from build123d import *

# Parameters (mm, degrees)
PAD009_DEPTH    = 350
POCKET015_DEPTH = 22.001
PAD010_DEPTH    = 20
SKETCH031_R     = 1.5
POCKET016_DEPTH = 5
SKETCH032_R     = 1.5
POCKET017_DEPTH = 5
SKETCH033_R     = 1.5
POCKET018_DEPTH = 5
SKETCH035_R     = 1.5
POCKET020_DEPTH = 5
SKETCH071_R     = 1.5
POCKET047_DEPTH = 5


with BuildPart() as part:
    # Sketch028 (on Face2 of Binder006) → Pad009 (new body)
    with BuildSketch(Plane(origin=(0, -0.1, 0), x_dir=(-1, 0, 0), z_dir=(0, 1, 0))):
        Polygon((-627, -343.2), (-627, 133.2535631324), (-605.051890377, 134.7636902715), (-605.051890377, 132.7636902715), (-625, 131.2535631324), (-625, -341.2), (-605, -341.2), (-605, -343.2), align=None)
    extrude(amount=PAD009_DEPTH)

    # Sketch029 (on Face2 of Pad009) → Pocket015 (cut, through all)
    with BuildSketch(Plane.YZ.offset(627)):
        Polygon((-0.1, -203.2), (195.0232253156, 134.7636902715), (-0.1, 134.7636902715), align=None)
    extrude(amount=-POCKET015_DEPTH, mode=Mode.SUBTRACT)

    # Sketch030 (on Face9 of Pocket015) → Pad010 (join)
    with BuildSketch(Plane(origin=(625, 0, 0), x_dir=(0, -1, 0), z_dir=(-1, 0, 0))):
        Polygon((0.1, -341.2), (0.1, -203.2), (-192.9966545674, 131.2535631324), (-194.9966545674, 131.2535631324), (-1.9, -203.2), (-1.9, -341.2), align=None)
    extrude(amount=PAD010_DEPTH)

    # Sketch031 (on Face2 of Binder006) → Pocket016 (cut)
    with BuildSketch(Plane(origin=(0, -0.1, 0), x_dir=(-1, 0, 0), z_dir=(0, 1, 0))):
        with Locations((-615, -213.2)):
            Circle(SKETCH031_R)
        with Locations((-616.35879, -273.2)):
            Circle(SKETCH031_R)
        with Locations((-615, -333.2)):
            Circle(SKETCH031_R)
    extrude(amount=POCKET016_DEPTH, mode=Mode.SUBTRACT)

    # Sketch032 (on Face6 of Pocket016) → Pocket017 (cut)
    with BuildSketch(Plane(origin=(0, 87.9131353872, -50.7566197735), x_dir=(1, 0, 0), z_dir=(0, -0.8660256282, 0.4999996113))):
        with Locations((615, -166.026408)):
            Circle(SKETCH032_R)
        with Locations((615, 17.070397)):
            Circle(SKETCH032_R)
        with Locations((615, 113.6188)):
            Circle(SKETCH032_R)
        with Locations((615, 200.167202)):
            Circle(SKETCH032_R)
        with Locations((615, -74.478005)):
            Circle(SKETCH032_R)
    extrude(amount=-POCKET017_DEPTH, mode=Mode.SUBTRACT)

    # Sketch033 (on Face10 of Pocket017) → Pocket018 (cut)
    with BuildSketch(Plane.XY.offset(-341.2)):
        with Locations((615, 11.9)):
            Circle(SKETCH033_R)
        with Locations((615, 93.9)):
            Circle(SKETCH033_R)
        with Locations((615, 175.9)):
            Circle(SKETCH033_R)
        with Locations((615, 267.9)):
            Circle(SKETCH033_R)
        with Locations((615, 339.9)):
            Circle(SKETCH033_R)
    extrude(amount=-POCKET018_DEPTH, mode=Mode.SUBTRACT)

    # Sketch035 (on Face19 of Pocket018) → Pocket020 (cut)
    with BuildSketch(Plane(origin=(12.0794992713, 0, 175.5628167535), x_dir=(0.9976413465, 0, -0.0686421427), z_dir=(0.0686421427, 0, 0.9976413465))):
        with Locations((604.374314, 272.461613)):
            Circle(SKETCH035_R)
        with Locations((604.374314, 339.9)):
            Circle(SKETCH035_R)
        with Locations((604.374314, 205.023225)):
            Circle(SKETCH035_R)
    extrude(amount=-POCKET020_DEPTH, mode=Mode.SUBTRACT)

    # Sketch071 (on Face1 of Binder021) → Pocket047 (cut)
    with BuildSketch(Plane.YZ.offset(629)):
        with Locations((339.9, -213.170471)):
            Circle(SKETCH071_R)
        with Locations((257.904262, -213.170471)):
            Circle(SKETCH071_R)
        with Locations((175.908524, -213.170471)):
            Circle(SKETCH071_R)
        with Locations((93.912786, -213.170471)):
            Circle(SKETCH071_R)
        with Locations((11.917049, -213.170471)):
            Circle(SKETCH071_R)
    extrude(amount=-POCKET047_DEPTH, mode=Mode.SUBTRACT)


solid = part.part
Source: CAD feature listing. Evaluate the final solid. Frame: model axes, mm. A direction names the side the tool comes from. Coordinates: 2 decimals unless noted, no trailing zeros. Order: outer loops, then holes, each group sorted by start corner. A loop starts at its lowest first (then second) coordinate and runs counter-clockwise, first axis right, second up. Notation, with made-up numbers: M 7.25,15 L 37.25,15 A26 ccw 37.25,39 Z; hole C 20.25,61.25 d5. An arc over 180 degrees is marked long. Write each question's results on one line, items separated by ' | '. Start each with the question number.
1. Pin query (flat end, axial travel): pin 1 (2.5 mm diameter, centred on x = 615, y = 93.9, fed in from -Z); pin 2 (4 mm diameter, centred on y = 339.9, z = -213.17, fed in from -X); pin 3 (4 mm diameter, centred on x = 615, y = 267.9, fed in from -Z); pin 4 (1 mm diameter, centred on x = 610.5, y = 193.5, fed in from +Z). Return the tip coordinate at first contact, or that it passes through.
2. Section A-A, the plane y = 237. Return the cut outline in (x, z).
3. Section B-B, the plane z = -92.5. Return the cut outline in (x, y), then the cut area to 3 significant figures.
4. Reachability of faces 1 (the face through (615, 173, -341.2)), 2 (the face through (614, -0.1, -274)) from +Z, -Z, +X, -X, +Y, -Y: full face, straight path, thin tool, end or side. Return the list, or none.
5. Material intervals for L1, parallel to Y at x = 615, z = -342; L2, parallel to Z at x = 615, y = 1.1; L3, parallel to Z at x = 615, y = 258, sorted ascending.
6. Draft query along Z for faces 3 (the face through (616.18, 270.94, 134)), 4 (the face through (625, 212, -154)), 5 (the face through (616, 172, -343.2)), 6 (the face through (627, 211, -161)). Return one class per face: +Z half, -Z half, draft (parallel to the pull), parting line (faces both ways), or undercut.
7. Section C-C, the plane y = 157. Return the cut outline in (x, z), then the cut area to 3 significant figures.
8. Section D-D, the plane z = -172. Return the cut outline in (x, y), then the cut area to 3 significant figures.
Solution:
1) pin 1: z = -46.02 | pin 2: x = 625 | pin 3: z = -343.2 | pin 4: z = 132.99
2) outline: M 605,-343.2 L 627,-343.2 L 627,133.25 L 605.05,134.76 L 605.05,132.76 L 625,131.25 L 625,-341.2 L 605,-341.2 Z
3) outline: M 605,63.81 L 627,63.81 L 627,349.9 L 625,349.9 L 625,65.81 L 605,65.81 Z | area: 612 mm²
4) face 1: -X, +Y | face 2: +Z, -Z, +X, -X, -Y
5) L1: -0.1 to 10.4, 13.4 to 92.4, 95.4 to 174.4, 177.4 to 266.4, 269.4 to 338.4, 341.4 to 349.9 | L2: -343.2 to -334.7, -331.7 to -273.84, -272.56 to -214.7, -211.7 to -201.12 | L3: -343.2 to -341.2, 132.01 to 134.08
6) face 3: +Z half | face 4: undercut | face 5: -Z half | face 6: draft
7) outline: M 605,-343.2 L 627,-343.2 L 627,68.91 L 605,68.91 L 605,65.44 L 625,65.44 L 625,-341.2 L 605,-341.2 Z | area: 933 mm²
8) outline: M 605,17.91 L 627,17.91 L 627,349.9 L 625,349.9 L 625,19.91 L 605,19.91 Z | area: 704 mm²
